from build123d import *

# Parameters (mm, degrees)
SKETCH1_W               = 90
SKETCH1_H               = 70
BOSS_EXTRUDE1_DEPTH     = 2
SKETCH2_W               = 90
SKETCH2_H               = 70
BOSS_EXTRUDE2_DEPTH     = 5
CUT_EXTRUDE2_START      = -2
SKETCH3_R               = 1.5
CUT_EXTRUDE2_DEPTH      = 5
SKETCH9_W               = 5
SKETCH9_H               = 70
BOSS_EXTRUDE6_DEPTH     = 2
SKETCH9_2_W             = 5
SKETCH9_2_H             = 70
BOSS_EXTRUDE7_DEPTH     = 30
SKETCH11_R              = 1.5
CUT_EXTRUDE6_DEPTH      = 69.007352544
CUT_EXTRUDE7_DEPTH      = 111.675200474
CUT_EXTRUDE7_DEPTH_BACK = 10
BOSS_EXTRUDE8_START     = -2
SKETCH12_W              = 29
SKETCH12_H              = 20
BOSS_EXTRUDE8_DEPTH     = 25
SKETCH13_W              = 25
SKETCH13_H              = 16
CUT_EXTRUDE8_DEPTH      = 25
SKETCH14_W              = 21.535675489
SKETCH14_H              = 27.087328124
SKETCH14_W_2            = 37.464324511
CUT_EXTRUDE9_DEPTH      = 25
SKETCH15_R              = 1.5
CUT_EXTRUDE10_DEPTH     = 25
BOSS_EXTRUDE9_START     = -3
SKETCH16_W              = 5
SKETCH16_H              = 70
BOSS_EXTRUDE9_DEPTH     = 3


with BuildPart() as part:
    # Sketch1 → Boss-Extrude1 (new body)
    with BuildSketch(Plane(origin=(0, 0, 0), x_dir=(1, 0, 0), z_dir=(0, 1, 0))):
        Rectangle(SKETCH1_W, SKETCH1_H)
    extrude(amount=BOSS_EXTRUDE1_DEPTH)

    # Sketch2 → Boss-Extrude2 (add)
    with BuildSketch(Plane(origin=(0, 2, 0), x_dir=(1, 0, 0), z_dir=(0, 1, 0))):
        Rectangle(SKETCH2_W, SKETCH2_H)
    extrude(amount=-BOSS_EXTRUDE2_DEPTH)

    # Sketch3 → Cut-Extrude2 (cut)
    with BuildSketch(Plane.XZ.offset(CUT_EXTRUDE2_START)):
        with Locations(Location((-40, 30, 0), (0, 0, 90))):
            Circle(SKETCH3_R)
        with Locations(Location((-19, 30, 0), (0, 0, 90))):
            Circle(SKETCH3_R)
        with Locations(Location((-4.5, 30, 0), (0, 0, 90))):
            Circle(SKETCH3_R)
        with Locations(Location((22.5, 30, 0), (0, 0, 90))):
            Circle(SKETCH3_R)
    extrude(amount=CUT_EXTRUDE2_DEPTH, mode=Mode.SUBTRACT)

    # Sketch9 → Boss-Extrude6 (add)
    with BuildSketch(Plane(origin=(0, 2, 0), x_dir=(1, 0, 0), z_dir=(0, 1, 0))):
        with Locations((-47.5, 0)):
            Rectangle(SKETCH9_W, SKETCH9_H)
        with Locations((47.5, 0)):
            Rectangle(SKETCH9_W, SKETCH9_H)
    extrude(amount=-BOSS_EXTRUDE6_DEPTH)

    # Sketch9<2> → Boss-Extrude7 (add)
    with BuildSketch(Plane(origin=(0, 2, 0), x_dir=(1, 0, 0), z_dir=(0, 1, 0))):
        with Locations((-47.5, 0)):
            Rectangle(SKETCH9_2_W, SKETCH9_2_H)
        with Locations((47.5, 0)):
            Rectangle(SKETCH9_2_W, SKETCH9_2_H)
    extrude(amount=BOSS_EXTRUDE7_DEPTH)

    # Sketch11 → Cut-Extrude6 (cut, through all)
    with BuildSketch(Plane(origin=(0, 2, 0), x_dir=(1, 0, 0), z_dir=(0, 1, 0))):
        with Locations(Location((-47.5, -32.049006617, 0), (0, 0, 270))):
            Circle(SKETCH11_R)
        with Locations(Location((-47.5, 32.049006617, 0), (0, 0, 90))):
            Circle(SKETCH11_R)
        with Locations(Location((47.5, 32.049006617, 0), (0, 0, 270))):
            Circle(SKETCH11_R)
        with Locations(Location((47.5, -32.049006617, 0), (0, 0, 90))):
            Circle(SKETCH11_R)
    extrude(amount=CUT_EXTRUDE6_DEPTH, mode=Mode.SUBTRACT)

    # Sketch10 → Cut-Extrude7 (cut, two sides: drawn at the far end of the back side and taken through both)
    with BuildSketch(Plane(origin=(50, 0, 0), x_dir=(0, 0, -1), z_dir=(1, 0, 0)).offset(-CUT_EXTRUDE7_DEPTH_BACK)):
        Polygon((-29.5, 26.895487084), (-29.5, 7.104512916), (-29.5, 4.912671876), (29.5, 4.912671876), (29.5, 29.087328124), (29.5, 32), (-29.5, 32), (-29.5, 29.087328124), align=None)
    extrude(amount=CUT_EXTRUDE7_DEPTH + CUT_EXTRUDE7_DEPTH_BACK, mode=Mode.SUBTRACT)

    # Sketch12 → Boss-Extrude8 (add)
    with BuildSketch(Plane.XZ.offset(BOSS_EXTRUDE8_START)):
        with Locations((-29.5, -24)):
            Rectangle(SKETCH12_W, SKETCH12_H)
    extrude(amount=-BOSS_EXTRUDE8_DEPTH)

    # Sketch13 → Cut-Extrude8 (cut)
    with BuildSketch(Plane(origin=(0, 27, 0), x_dir=(-1, 0, 0), z_dir=(0, 1, 0))):
        with Locations((29.5, -24)):
            Rectangle(SKETCH13_W, SKETCH13_H)
    extrude(amount=-CUT_EXTRUDE8_DEPTH, mode=Mode.SUBTRACT)

    # Sketch14 → Cut-Extrude9 (cut)
    with BuildSketch(Plane(origin=(-45, 0, 0), x_dir=(0, 0, -1), z_dir=(1, 0, 0))):
        with Locations((24.232162256, 18.456335938)):
            Rectangle(SKETCH14_W, SKETCH14_H)
        with Locations((-10.767837745, 18.456335938)):
            Rectangle(SKETCH14_W_2, SKETCH14_H)
    extrude(amount=-CUT_EXTRUDE9_DEPTH, mode=Mode.SUBTRACT)

    # Sketch15 → Cut-Extrude10 (cut)
    with BuildSketch(Plane(origin=(0, 32, 0), x_dir=(1, 0, 0), z_dir=(0, 1, 0))):
        with Locations(Location((-47.5, 10.653576943, 0), (0, 0, 270))):
            Circle(SKETCH15_R)
    extrude(amount=-CUT_EXTRUDE10_DEPTH, mode=Mode.SUBTRACT)

    # Sketch16 → Boss-Extrude9 (add)
    with BuildSketch(Plane.XZ.offset(3).offset(BOSS_EXTRUDE9_START)):
        with Locations((-47.5, 0)):
            Rectangle(SKETCH16_W, SKETCH16_H)
        with Locations((47.5, 0)):
            Rectangle(SKETCH16_W, SKETCH16_H)
    extrude(amount=BOSS_EXTRUDE9_DEPTH)


solid = part.part
Source: CAD feature listing. Evaluate the final solid. Frame: model axes, mm. A direction names the side the tool comes from. Coordinates: 2 decimals unless noted, no trailing zeros. Loops run counter-clockwise (first coordinate to the right, second up) from the corner with the lowest first, then second, coordinate; pieces in that order, holes last. Notation, with made-up numbers: M -32,23 L 6,23 A11 ccw 6,37 Z; hole C 38,12 d3. An arc over 180 degrees is marked long. Answer in a Markdown table with one row per item.
Q1. Set-up query: faces 1 (the flat face through (-47, 4.913, -24)), 2 (the flat face through (-47, 7, -11)), 3 (the flat face through (45, 4.7, 0.2)). Return all of +Z, -Z, +X, -X, +Y, -Y with unobstructed straight access to the full face (end or side cutting, diameter ignored); none if empty.
Answers below:
| item | result |
|---|---|
| face 1 | -Z, -X, +Y |
| face 2 | +Y |
| face 3 | +Z, -Z, +Y |
Q2. Section A-A on y = 19. State how many separate pieces and enclosed holes the cut face has, plus the area to 3 significant figures.
Answers below:
| item | result |
|---|---|
| separate pieces | 5 |
| enclosed holes | 5 |
| area | 262 mm^2 |
Q3. Draft query along X for faces 4 (the flat face through (-42, 15, -24)), 5 (the flat face through (-49, 32, 33)), 6 (the flat face through (50, 3, 0)). Return one class per face: pulls with the +X half, pulls with the -X half, needs draft (parallel to the pull), parting line crosses it, or undercut.
Answers below:
| item | result |
|---|---|
| face 4 | undercut |
| face 5 | needs draft |
| face 6 | pulls with the +X half |
Q4. Section C-C on z = 3. Return the cut outline in (x, y), plus the area to 3 significant figures.
Answers below:
| item | result |
|---|---|
| outline | M -50,-3 L 50,-3 L 50,4.91 L 45,4.91 L 45,2 L -45,2 L -45,4.91 L -50,4.91 Z |
| area | 529 mm^2 |
Q5. Section B-B on x = -19. Return the cut outline in (y, z).
Answers below:
| item | result |
|---|---|
| outline | M -3,-35 L 2,-35 L 2,-34 L 27,-34 L 27,-32 L 2,-32 L 2,-16 L 27,-16 L 27,-14 L 2,-14 L 2,28.5 L -3,28.5 Z; M -3,31.5 L 2,31.5 L 2,35 L -3,35 Z |
Q6. Section D-D on x = -34. Return the cut outline in (y, z).
Answers below:
| item | result |
|---|---|
| outline | M -3,-35 L 2,-35 L 2,-34 L 27,-34 L 27,-32 L 2,-32 L 2,-16 L 27,-16 L 27,-14 L 2,-14 L 2,35 L -3,35 Z |
Q7. Ray query, probe 1 along X at (y, z) = (-0.2, 30); probe 2 along Z at (x, y) = (-38, 11.5); probe 3 along Z at (x, y) = (47, 10). Return the intervals inside material, ascending. Write a range as from..to.
Answers below:
| item | result |
|---|---|
| probe 1 | x = -50..-41.5, -38.5..-20.5, -17.5..-6, -3..21, 24..50 |
| probe 2 | z = -34..-32, -16..-14 |
| probe 3 | z = -35..-33.46, -30.63..-29.5, 29.5..30.63, 33.46..35 |
Q8. First-contact query: pin 1 (1 mm diameter, centred on x = 26, z = 10.5, fed in from +Y); pin 2 (12.5 mm diameter, centred on x = -29.5, y = 10, fed in from -Z); pin 3 (5 mm diameter, centred on y = 8, z = -17.5, fed in from +X). Flat tips, straight axial feed; report the tip coordinate or a pass-through.
Answers below:
| item | result |
|---|---|
| pin 1 | stops at y = 2 |
| pin 2 | stops at z = -34 |
| pin 3 | stops at x = -15 |
